Input: part model. Units: mm. Frame: model coordinates. Face numbers are marked on the shaded views. A direction names the side the tool comes from. Coordinates: 2 decimals unless noted, no trailing zeros. Order: outer loops, then holes, each group sorted by start corner. A loop starts at its lowest first (then second) coordinate and runs counter-clockwise, first axis right, second up. Notation, with made-up numbers: M 52,-12 L 74,-12 A24 ccw 74,24 Z; hole C 49.25,-38 d7. An arc over 180 degrees is marked long. Answer in a Markdown table with one row per item.
from build123d import *

# Parameters (mm, degrees)
SKETCH_1_W          = 8.2
SKETCH_1_H          = 4.2
EXTRUDE_1_DEPTH     = 18
SKETCH_2_W          = 13
SKETCH_2_H          = 9
SKETCH_2_W_2        = 8.2
SKETCH_2_H_2        = 4.2
EXTRUDE_2_DEPTH     = 3.7
FILLET_1_R          = 1
FILLET_2_R          = 0.3
EXTRUDE_3_DEPTH     = 0.2
CUT_EXTRUDE_1_DEPTH = 10
FILLET_3_R          = 0.3


with BuildPart() as part:
    # 草图1 → 凸台-拉伸1 (new body)
    with BuildSketch(Plane(origin=(0, 0, 0), x_dir=(1, 0, 0), z_dir=(0, 1, 0))):
        with Locations((11.994336416, 2.5)):
            Rectangle(SKETCH_1_W, SKETCH_1_H)
    extrude(amount=EXTRUDE_1_DEPTH)

    # 草图2 → 凸台-拉伸2 (add)
    with BuildSketch(Plane.XZ):
        with Locations((11.994336416, -2.5)):
            Rectangle(SKETCH_2_W, SKETCH_2_H)
        with Locations((11.994336416, -2.5)):
            Rectangle(SKETCH_2_W_2, SKETCH_2_H_2, mode=Mode.SUBTRACT)
    extrude(amount=-EXTRUDE_2_DEPTH)

    # 圆角1
    fillet_1_edges = [part.edges().sort_by_distance(p)[0] for p in [
        (7.894336416, 10.85, -4.6),
        (16.094336416, 10.85, -4.6),
        (16.094336416, 10.85, -0.4),
        (7.894336416, 10.85, -0.4),
    ]]
    fillet(fillet_1_edges, radius=FILLET_1_R)

    # 圆角2
    fillet_2_edges = [part.edges().sort_by_distance(p)[0] for p in [
        (11.994336416, 3.7, 2),
        (5.494336416, 1.85, 2),
        (18.494336416, 3.7, -2.5),
        (18.494336416, 1.85, 2),
        (11.994336416, 3.7, -7),
        (18.494336416, 1.85, -7),
        (5.494336416, 3.7, -2.5),
        (5.494336416, 1.85, -7),
        (11.994336416, 18, -4.6),
        (16.094336416, 18, -2.5),
        (7.894336416, 18, -2.5),
        (11.994336416, 18, -0.4),
        (8.187229635, 18, -0.692893219),
        (8.187229635, 18, -4.307106781),
        (15.801443197, 18, -0.692893219),
        (15.801443197, 18, -4.307106781),
    ]]
    fillet(fillet_2_edges, radius=FILLET_2_R)

    # 草图3 → 凸台-拉伸3 (add)
    with BuildSketch(Plane(origin=(0, 18, 0), x_dir=(1, 0, 0), z_dir=(0, 1, 0))):
        Polygon((11.994336416, 2.5), (12.194336416, 2.5), (12.194336416, 4.3), (11.794336416, 4.3), (11.794336416, 2.5), align=None)
        with BuildLine():
            Line((11.594336416, 3.416515139), (11.594336416, 3.945683229))
            ThreePointArc((11.594336416, 3.945683229), (11.994336416, 1), (12.394336416, 3.945683229))
            Line((12.394336416, 3.945683229), (12.394336416, 3.416515139))
            ThreePointArc((12.394336416, 3.416515139), (11.994336416, 1.5), (11.594336416, 3.416515139))
        make_face()
    extrude(amount=EXTRUDE_3_DEPTH)

    # 草图4 → 切除-拉伸1 (cut)
    with BuildSketch(Plane(origin=(0, 3.7, 0), x_dir=(1, 0, 0), z_dir=(0, 1, 0))):
        Polygon((11.994336416, 0.4), (4.788962203, 0.4), (4.788962203, -2.393061312), (19.340992476, -2.393061312), (19.340992476, 0.4), align=None)
    extrude(amount=-CUT_EXTRUDE_1_DEPTH, mode=Mode.SUBTRACT)

    # 圆角3
    fillet_3_edges = [part.edges().sort_by_distance(p)[0] for p in [
        (18.40646845, 3.612132034, -0.4),
        (5.494336416, 0, -3.55),
        (5.582204382, 3.612132034, -0.4),
        (5.494336416, 1.7, -0.4),
        (18.494336416, 1.7, -0.4),
        (11.994336416, 0, -0.4),
        (16.644336416, 3.7, -0.4),
        (7.344336416, 3.7, -0.4),
        (18.494336416, 0, -3.55),
        (11.994336416, 0, -7),
        (5.582204382, 0, -6.912132034),
        (18.40646845, 0, -6.912132034),
    ]]
    fillet(fillet_3_edges, radius=FILLET_3_R)


solid = part.part
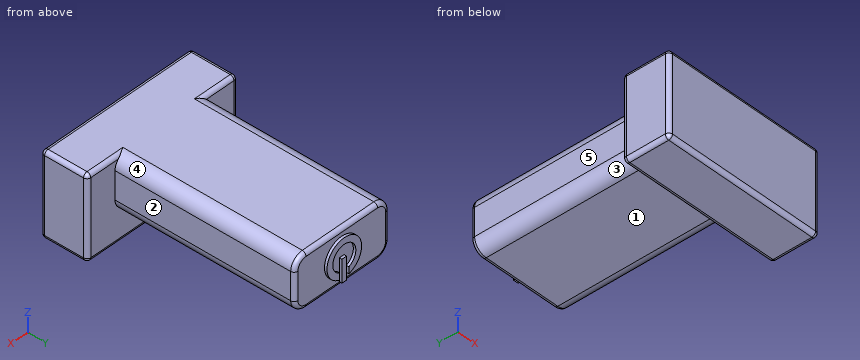
1) Material intervals for probe 1 along Z at (x, y) = (14.25, 11.5); probe 2 along Y at (x, z) = (8.75, -2); probe 3 along Y at (x, z) = (17.5, -5.25), sorted ascending.
Resolved:
| item | result |
|---|---|
| probe 1 | z = -4.6 to -0.4 |
| probe 2 | y = 0 to 18 |
| probe 3 | y = 0 to 3.7 |
2) Contact query for flat-ended pins moving along their axis: pin 1 (1.9 mm diameter, centred on x = 12.5, y = 9.5, fed in from -Z); pin 2 (2.5 mm diameter, centred on y = 13, z = -3, fed in from +X); pin 3 (0.7 mm diameter, centred on y = 9, z = -2, fed in from -X). Output: stop coordinate, or through.
Resolved:
| item | result |
|---|---|
| pin 1 | stops at z = -4.6 |
| pin 2 | stops at x = 16.09 |
| pin 3 | stops at x = 7.89 |
3) Cut plane B-B, the plane y = 17.25. Output: boundary loops of the cut face in (x, z).
Resolved:
| item | result |
|---|---|
| outline | M 7.89,-3.6 A1 ccw 8.89,-4.6 L 15.09,-4.6 A1 ccw 16.09,-3.6 L 16.09,-1.4 A1 ccw 15.09,-0.4 L 8.89,-0.4 A1 ccw 7.89,-1.4 Z |
4) Reachability of the marked faces 1, 2, 3, 4 and 5 from +Z, -Z, +X, -X, +Y, -Y: full face, straight path, thin tool, end or side. Return the list, or none.
Resolved:
| item | result |
|---|---|
| face 1 | -Z, +X, -X, +Y |
| face 2 | +Z, -Z, +X, +Y |
| face 3 | -Z, -X, +Y |
| face 4 | +Z, +X, +Y |
| face 5 | +Z, -Z, -X, +Y |
5) Cut plane D-D, the plane x = 17. Output: boundary loops of the cut face in (y, z), and give its area (3 significant figures).
Resolved:
| item | result |
|---|---|
| outline | M 0,-6.7 A0.3 ccw 0.3,-7 L 3.4,-7 A0.3 ccw 3.7,-6.7 L 3.7,-0.7 A0.3 ccw 3.4,-0.4 L 0.3,-0.4 A0.3 ccw 0,-0.7 Z |
| area | 24.3 mm2 |
6) Cut plane C-C, the plane z = -2.75. Output: boundary loops of the cut face in (x, y).
Resolved:
| item | result |
|---|---|
| outline | M 5.49,0.3 A0.3 ccw 5.79,0 L 18.19,0 A0.3 ccw 18.49,0.3 L 18.49,3.4 A0.3 ccw 18.19,3.7 L 16.09,3.7 L 16.09,17.7 A0.3 ccw 15.79,18 L 13.47,18 L 13.47,18.2 L 12.96,18.2 L 12.96,18 L 12.19,18 L 12.19,18.2 L 11.79,18.2 L 11.79,18 L 11.03,18 L 11.03,18.2 L 10.52,18.2 L 10.52,18 L 8.19,18 A0.3 ccw 7.89,17.7 L 7.89,3.7 L 5.79,3.7 A0.3 ccw 5.49,3.4 Z |
7) Cut plane A-A, the plane x = 13.75. Output: boundary loops of the cut face in (y, z).
Resolved:
| item | result |
|---|---|
| outline | M 0,-6.7 A0.3 ccw 0.3,-7 L 3.4,-7 A0.3 ccw 3.7,-6.7 L 3.7,-4.6 L 17.7,-4.6 A0.3 ccw 18,-4.3 L 18,-0.7 A0.3 ccw 17.7,-0.4 L 0.3,-0.4 A0.3 ccw 0,-0.7 Z |
